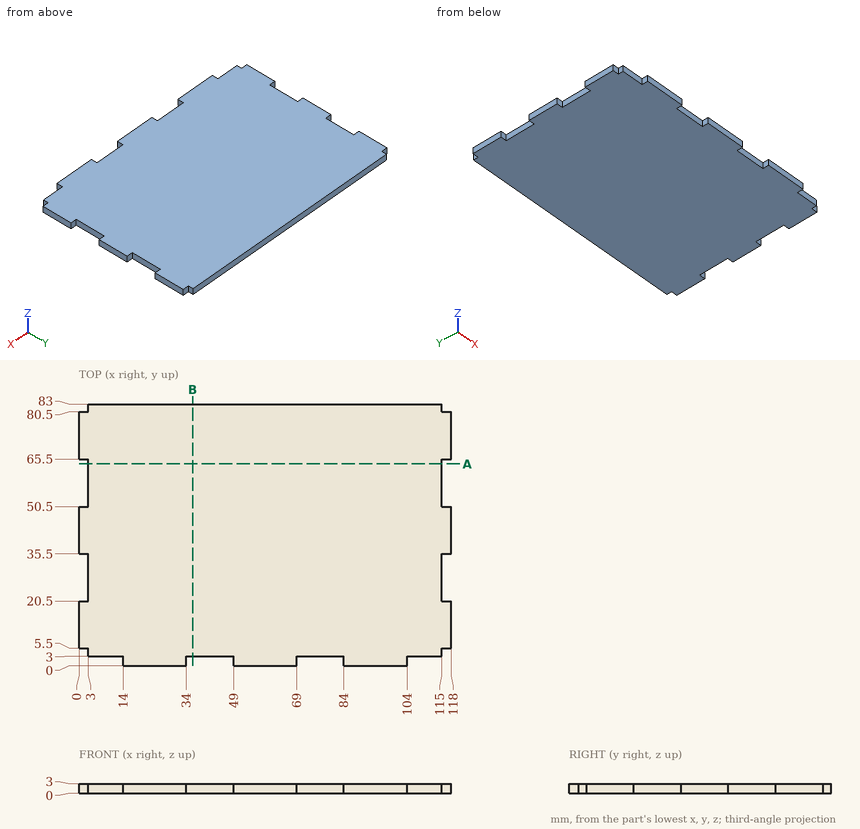
Answer from the drawing. Dimensions are ordinates in mm from the lowest x, y and z of the part. Coordinates: 2 decimals unless noted, no trailing zeros. Write each loop counter-clockwise with the first axis right and the second up, starting at its lowest first coordinate (ties: lowest second). Pieces come first, ordered by that corner, then holes. Notation, with made-up numbers: (-29, -28.5) - (15, -28.5) arc R15 ccw to (15, -17.5) - close; hole circle Ø4 at (9, -13). An arc over 180 degrees is marked (long way). One line per question, with ' | ' between items.
Q1. Find section B-B, the plane x = 36. Write down the section's boundary in (y, z).
Result set:
outline: (3, 0) - (83, 0) - (83, 3) - (3, 3) - close
Q2. Find section A-A, the plane y = 64. Write down the section's boundary in (x, z).
Result set:
outline: (3, 0) - (115, 0) - (115, 3) - (3, 3) - close
Q3. Each of these flat-tipped pins is pushed along its axis until it touches: P1, Ø1.5, axis at y = 1, z = 2, coming from the +X side; P2, Ø0.8, axis at y = 81.5, z = 1, coming from the -X side; P3, Ø1.2, axis at y = 4, z = 2, coming from the +X side; P4, Ø4, axis at x = 51, y = 42.5, coming from the -Z side. Where does it stop, or does it pass through?
Result set:
P1: x = 104 | P2: x = 3 | P3: x = 115 | P4: z = 0
Q4. Consider L1, parallel to X at y = 23, z = 2.15; L2, parallel to Y at x = 44.5, z = 0.2. Determine where each line is inside the solid, lowest interval first. Write a range as [from, to].
Result set:
L1: [3, 115] | L2: [3, 83]
